Check sheet for the modelled part. Datum: model origin and axes. Units: mm. Round coordinates to 2 decimals unless told otherwise and drop trailing zeros. Write each loop counter-clockwise with the first axis right and the second up, starting at its lowest first coordinate (ties: lowest second). Pieces come first, ordered by that corner, then holes. Notation, with made-up numbers: M 23.25,58 L 80.25,58 A13 cw 80.25,72 Z; hole C -7.5,21 d8. An arc over 180 degrees is marked long. Put each result on its own line as item: value.
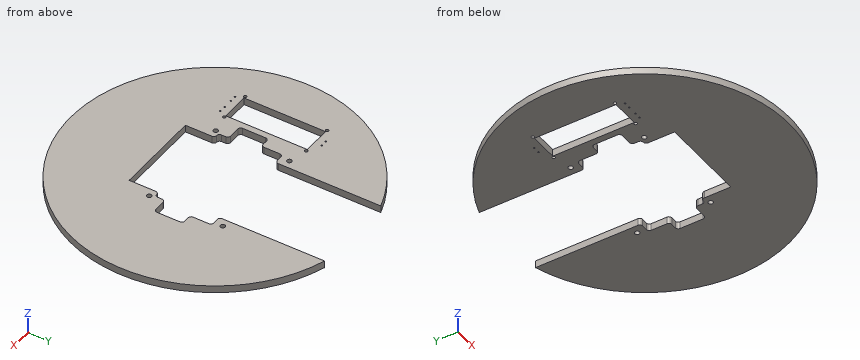
```python
from build123d import *

# Parameters (mm, degrees)
BOSS_EXTRUDE1_DEPTH = 6.35
CUT_EXTRUDE1_REACH  = 210.789
SKETCH2_R           = 1.3335
SKETCH2_W           = 24.765
SKETCH2_H           = 71.755
CUT_EXTRUDE2_REACH  = 210.789
SKETCH3_R           = 0.635
CUT_EXTRUDE3_DEPTH  = 209.788828163
FILLET1_START       = -1
FILLET1_DEPTH       = 8
FILLET1_2_DEPTH     = 6.35
SKETCH5_R           = 2.0828
CUT_EXTRUDE4_DEPTH  = 209.788828163


with BuildPart() as part:
    # Sketch1 → Boss-Extrude1 (new body)
    with BuildSketch(Plane.XY):
        with BuildLine():
            Line((-38.1, 92.71), (-38.1, 165.60027858))
            ThreePointArc((-38.1, 165.60027858), (0, -82.55), (38.1, 165.60027858))
            Line((38.1, 165.60027858), (38.1, 92.71))
            Line((38.1, 92.71), (38.1, -6.35))
            Line((38.1, -6.35), (-38.1, -6.35))
            Line((-38.1, -6.35), (-38.1, 92.71))
        make_face()
    extrude(amount=BOSS_EXTRUDE1_DEPTH)

    # Sketch2 → Cut-Extrude1 (cut, up to next)
    with BuildSketch(Plane(origin=(0, 0, 0), x_dir=(-1, 0, 0), z_dir=(0, 0, -1)), mode=Mode.PRIVATE) as cut_extrude1_sk1:
        with Locations((61.7855, 12.5095)):
            Circle(SKETCH2_R)
    cut_extrude1_tool1 = extrude(cut_extrude1_sk1.sketch, amount=-CUT_EXTRUDE1_REACH, mode=Mode.PRIVATE) & part.part
    # Sketch2 → Cut-Extrude1 (cut, up to next)
    with BuildSketch(Plane(origin=(0, 0, 0), x_dir=(-1, 0, 0), z_dir=(0, 0, -1)), mode=Mode.PRIVATE) as cut_extrude1_sk2:
        with Locations((61.7855, 84.6455)):
            Circle(SKETCH2_R)
    cut_extrude1_tool2 = extrude(cut_extrude1_sk2.sketch, amount=-CUT_EXTRUDE1_REACH, mode=Mode.PRIVATE) & part.part
    # Sketch2 → Cut-Extrude1 (cut, up to next)
    with BuildSketch(Plane(origin=(0, 0, 0), x_dir=(-1, 0, 0), z_dir=(0, 0, -1)), mode=Mode.PRIVATE) as cut_extrude1_sk3:
        with Locations((89.9795, 84.6455)):
            Circle(SKETCH2_R)
    cut_extrude1_tool3 = extrude(cut_extrude1_sk3.sketch, amount=-CUT_EXTRUDE1_REACH, mode=Mode.PRIVATE) & part.part
    # Sketch2 → Cut-Extrude1 (cut, up to next)
    with BuildSketch(Plane(origin=(0, 0, 0), x_dir=(-1, 0, 0), z_dir=(0, 0, -1)), mode=Mode.PRIVATE) as cut_extrude1_sk4:
        with Locations((89.9795, 12.5095)):
            Circle(SKETCH2_R)
    cut_extrude1_tool4 = extrude(cut_extrude1_sk4.sketch, amount=-CUT_EXTRUDE1_REACH, mode=Mode.PRIVATE) & part.part
    # Sketch2 → Cut-Extrude1 (cut, up to next)
    with BuildSketch(Plane(origin=(0, 0, 0), x_dir=(-1, 0, 0), z_dir=(0, 0, -1)), mode=Mode.PRIVATE) as cut_extrude1_sk5:
        with Locations((75.8825, 48.5775)):
            Rectangle(SKETCH2_W, SKETCH2_H)
    cut_extrude1_tool5 = extrude(cut_extrude1_sk5.sketch, amount=-CUT_EXTRUDE1_REACH, mode=Mode.PRIVATE) & part.part
    add(cut_extrude1_tool1.solids().sort_by_distance((-61.7855, 12.5095, 0))[0], mode=Mode.SUBTRACT)
    add(cut_extrude1_tool2.solids().sort_by_distance((-61.7855, 84.6455, 0))[0], mode=Mode.SUBTRACT)
    add(cut_extrude1_tool3.solids().sort_by_distance((-89.9795, 84.6455, 0))[0], mode=Mode.SUBTRACT)
    add(cut_extrude1_tool4.solids().sort_by_distance((-89.9795, 12.5095, 0))[0], mode=Mode.SUBTRACT)
    add(cut_extrude1_tool5.solids().sort_by_distance((-75.8825, 48.5775, 0))[0], mode=Mode.SUBTRACT)

    # Sketch3 → Cut-Extrude2 (cut, up to next)
    with BuildSketch(Plane.XY.offset(6.35), mode=Mode.PRIVATE) as cut_extrude2_sk1:
        with Locations((-66.04, 6.35)):
            Circle(SKETCH3_R)
    cut_extrude2_tool1 = extrude(cut_extrude2_sk1.sketch, amount=-CUT_EXTRUDE2_REACH, mode=Mode.PRIVATE) & part.part
    # Sketch3 → Cut-Extrude2 (cut, up to next)
    with BuildSketch(Plane.XY.offset(6.35), mode=Mode.PRIVATE) as cut_extrude2_sk2:
        with Locations((-71.628, 6.35)):
            Circle(SKETCH3_R)
    cut_extrude2_tool2 = extrude(cut_extrude2_sk2.sketch, amount=-CUT_EXTRUDE2_REACH, mode=Mode.PRIVATE) & part.part
    # Sketch3 → Cut-Extrude2 (cut, up to next)
    with BuildSketch(Plane.XY.offset(6.35), mode=Mode.PRIVATE) as cut_extrude2_sk3:
        with Locations((-80.137, 6.35)):
            Circle(SKETCH3_R)
    cut_extrude2_tool3 = extrude(cut_extrude2_sk3.sketch, amount=-CUT_EXTRUDE2_REACH, mode=Mode.PRIVATE) & part.part
    # Sketch3 → Cut-Extrude2 (cut, up to next)
    with BuildSketch(Plane.XY.offset(6.35), mode=Mode.PRIVATE) as cut_extrude2_sk4:
        with Locations((-85.725, 6.35)):
            Circle(SKETCH3_R)
    cut_extrude2_tool4 = extrude(cut_extrude2_sk4.sketch, amount=-CUT_EXTRUDE2_REACH, mode=Mode.PRIVATE) & part.part
    # Sketch3 → Cut-Extrude2 (cut, up to next)
    with BuildSketch(Plane.XY.offset(6.35), mode=Mode.PRIVATE) as cut_extrude2_sk5:
        with Locations((-73.0885, 90.805)):
            Circle(SKETCH3_R)
    cut_extrude2_tool5 = extrude(cut_extrude2_sk5.sketch, amount=-CUT_EXTRUDE2_REACH, mode=Mode.PRIVATE) & part.part
    # Sketch3 → Cut-Extrude2 (cut, up to next)
    with BuildSketch(Plane.XY.offset(6.35), mode=Mode.PRIVATE) as cut_extrude2_sk6:
        with Locations((-78.6765, 90.805)):
            Circle(SKETCH3_R)
    cut_extrude2_tool6 = extrude(cut_extrude2_sk6.sketch, amount=-CUT_EXTRUDE2_REACH, mode=Mode.PRIVATE) & part.part
    add(cut_extrude2_tool1.solids().sort_by_distance((-66.04, 6.35, 6.35))[0], mode=Mode.SUBTRACT)
    add(cut_extrude2_tool2.solids().sort_by_distance((-71.628, 6.35, 6.35))[0], mode=Mode.SUBTRACT)
    add(cut_extrude2_tool3.solids().sort_by_distance((-80.137, 6.35, 6.35))[0], mode=Mode.SUBTRACT)
    add(cut_extrude2_tool4.solids().sort_by_distance((-85.725, 6.35, 6.35))[0], mode=Mode.SUBTRACT)
    add(cut_extrude2_tool5.solids().sort_by_distance((-73.0885, 90.805, 6.35))[0], mode=Mode.SUBTRACT)
    add(cut_extrude2_tool6.solids().sort_by_distance((-78.6765, 90.805, 6.35))[0], mode=Mode.SUBTRACT)

    # Sketch4 → Cut-Extrude3 (cut, through all)
    with BuildSketch(Plane.XY.offset(6.35)):
        Polygon((-48.26, 72.898), (-48.26, 53.848), (-58.1, 53.848), (-58.1, 28.448), (-43.18, 28.448), (-43.18, 19.558), (-38.1, 19.558), (-38.1, 72.898), align=None)
        Polygon((43.18, 28.448), (58.1, 28.448), (58.1, 53.848), (48.26, 53.848), (48.26, 72.898), (38.1, 72.898), (38.1, 19.558), (43.18, 19.558), align=None)
    extrude(amount=-CUT_EXTRUDE3_DEPTH, mode=Mode.SUBTRACT)

    # Fillet1: read off the stored shape, not the designer's step
    # Fillet1 outline → Fillet1 (cut)
    with BuildSketch(Plane.XY.offset(FILLET1_START)):
        with BuildLine():
            Line((38.1, 72.898), (40.64, 72.898))
            ThreePointArc((40.64, 72.898), (38.843948776, 73.641948776), (38.1, 75.438))
            Line((38.1, 75.438), (38.1, 72.898))
        make_face()
        with BuildLine():
            Line((48.26, 53.848), (50.8, 53.848))
            ThreePointArc((50.8, 53.848), (49.003948776, 54.591948776), (48.26, 56.388))
            Line((48.26, 56.388), (48.26, 53.848))
        make_face()
        with BuildLine():
            Line((43.18, 28.448), (43.18, 25.908))
            ThreePointArc((43.18, 25.908), (43.923948776, 27.704051224), (45.72, 28.448))
            Line((45.72, 28.448), (43.18, 28.448))
        make_face()
        with BuildLine():
            ThreePointArc((38.1, 17.018), (38.843948776, 18.814051224), (40.64, 19.558))
            Line((40.64, 19.558), (38.1, 19.558))
            Line((38.1, 19.558), (38.1, 17.018))
        make_face()
        with BuildLine():
            Line((-38.1, 19.558), (-40.64, 19.558))
            ThreePointArc((-40.64, 19.558), (-38.843948776, 18.814051224), (-38.1, 17.018))
            Line((-38.1, 17.018), (-38.1, 19.558))
        make_face()
        with BuildLine():
            ThreePointArc((-38.1, 75.438), (-38.843948776, 73.641948776), (-40.64, 72.898))
            Line((-40.64, 72.898), (-38.1, 72.898))
            Line((-38.1, 72.898), (-38.1, 75.438))
        make_face()
        with BuildLine():
            ThreePointArc((-48.26, 56.388), (-49.003948776, 54.591948776), (-50.8, 53.848))
            Line((-50.8, 53.848), (-48.26, 53.848))
            Line((-48.26, 53.848), (-48.26, 56.388))
        make_face()
        with BuildLine():
            ThreePointArc((-45.72, 28.448), (-43.923948776, 27.704051224), (-43.18, 25.908))
            Line((-43.18, 25.908), (-43.18, 28.448))
            Line((-43.18, 28.448), (-45.72, 28.448))
        make_face()
    extrude(amount=FILLET1_DEPTH, mode=Mode.SUBTRACT)

    # Fillet1 2 outline → Fillet1 2 (add)
    with BuildSketch(Plane.XY):
        with BuildLine():
            Line((43.18, 19.558), (43.18, 22.098))
            ThreePointArc((43.18, 22.098), (42.436051224, 20.301948776), (40.64, 19.558))
            Line((40.64, 19.558), (43.18, 19.558))
        make_face()
        with BuildLine():
            ThreePointArc((45.72, 72.898), (47.516051224, 72.154051224), (48.26, 70.358))
            Line((48.26, 70.358), (48.26, 72.898))
            Line((48.26, 72.898), (45.72, 72.898))
        make_face()
        with BuildLine():
            ThreePointArc((55.56, 53.848), (57.356051224, 53.104051224), (58.1, 51.308))
            Line((58.1, 51.308), (58.1, 53.848))
            Line((58.1, 53.848), (55.56, 53.848))
        make_face()
        with BuildLine():
            ThreePointArc((58.1, 30.988), (57.356051224, 29.191948776), (55.56, 28.448))
            Line((55.56, 28.448), (58.1, 28.448))
            Line((58.1, 28.448), (58.1, 30.988))
        make_face()
        with BuildLine():
            Line((-43.18, 19.558), (-40.64, 19.558))
            ThreePointArc((-40.64, 19.558), (-42.436051224, 20.301948776), (-43.18, 22.098))
            Line((-43.18, 22.098), (-43.18, 19.558))
        make_face()
        with BuildLine():
            Line((-48.26, 72.898), (-48.26, 70.358))
            ThreePointArc((-48.26, 70.358), (-47.516051224, 72.154051224), (-45.72, 72.898))
            Line((-45.72, 72.898), (-48.26, 72.898))
        make_face()
        with BuildLine():
            Line((-58.1, 53.848), (-58.1, 51.308))
            ThreePointArc((-58.1, 51.308), (-57.356051224, 53.104051224), (-55.56, 53.848))
            Line((-55.56, 53.848), (-58.1, 53.848))
        make_face()
        with BuildLine():
            Line((-58.1, 28.448), (-55.56, 28.448))
            ThreePointArc((-55.56, 28.448), (-57.356051224, 29.191948776), (-58.1, 30.988))
            Line((-58.1, 30.988), (-58.1, 28.448))
        make_face()
    extrude(amount=FILLET1_2_DEPTH)

    # Sketch5 → Cut-Extrude4 (cut, through all)
    with BuildSketch(Plane.XY.offset(6.35)):
        with Locations((-45.085, 80.645)):
            Circle(SKETCH5_R)
        with Locations(Location((45.085, 80.645, 0), (0, 0, 180))):
            Circle(SKETCH5_R)
        with Locations((45.085, 15.875)):
            Circle(SKETCH5_R)
        with Locations(Location((-45.085, 15.875, 0), (0, 0, 180))):
            Circle(SKETCH5_R)
    extrude(amount=-CUT_EXTRUDE4_DEPTH, mode=Mode.SUBTRACT)


solid = part.part
```
1. Depth check by flat-ended pin: pin 1 Ø3 at (y, z) = (-17, 1) entering from +X; pin 2 Ø3 at (y, z) = (101, 4.5) entering from +X; pin 3 Ø2.5 at (x, z) = (43.5, 4.5) entering from -Y. Enter the tip coordinate at first touch or a pass-through.
Computed values:
pin 1: stops at x = 111.96
pin 2: stops at x = 114.45
pin 3: stops at y = -75.32
2. Cross-section at A-A (y = 44.45). Enter the section's corners in (x, z) (3 decimals).
Computed values:
outline: M -127,0 L -88.265,0 L -88.265,6.35 L -127,6.35 Z; M -63.5,0 L -58.1,0 L -58.1,6.35 L -63.5,6.35 Z; M 58.1,0 L 127,0 L 127,6.35 L 58.1,6.35 Z
3. Cross-section at D-D (z = 3.5). Count the separate pieces of the cut face and the enclosed holes in it, then the cut area to 3 significant figures.
Computed values:
separate pieces: 1
enclosed holes: 15
area: 33,900 mm2
4. Scan lines: probe 1 along X at (y, z) = (91, 0.75); probe 2 along X at (y, z) = (56.5, 2.5) (3 decimals); probe 3 along Y at (x, z) = (1.5, 0.5). Record each from-to range of solid material in increasing order.
Computed values:
probe 1: x = -118.16 to -79.28, -78.07 to -73.69, -72.48 to -38.1, 38.1 to 118.16
probe 2: x = -126.427 to -88.265, -63.5 to -48.26, 48.26 to 126.427
probe 3: y = -82.54 to -6.35
5. Cross-section at C-C (x = 0). Enter the section's corners in (y, z).
Computed values:
outline: M -82.55,0 L -6.35,0 L -6.35,6.35 L -82.55,6.35 Z
6. Cross-section at B-B (y = 98). Enter the section's corners in (x, z), then the cut area to 3 significant figures.
Computed values:
outline: M -115.16,0 L -38.1,0 L -38.1,6.35 L -115.16,6.35 Z; M 38.1,0 L 115.16,0 L 115.16,6.35 L 38.1,6.35 Z
area: 979 mm2
